Check sheet for the drawn part. Datum: minimum x, y, z corner. Units: mm. Round coordinates to 2 decimals unless told otherwise and drop trailing zeros. Order: outer loops, then holes, each group sorted by start corner. A loop starts at its lowest first (then second) coordinate and runs counter-clockwise, first axis right, second up. Notation, with made-up numbers: (82, 66) - (140, 66) arc R17 cw to (140, 76) - close; hole circle Ø10 at (77.25, 84). An arc over 180 degrees is marked (long way). Write each question's results on one line, items separated by ' | '.
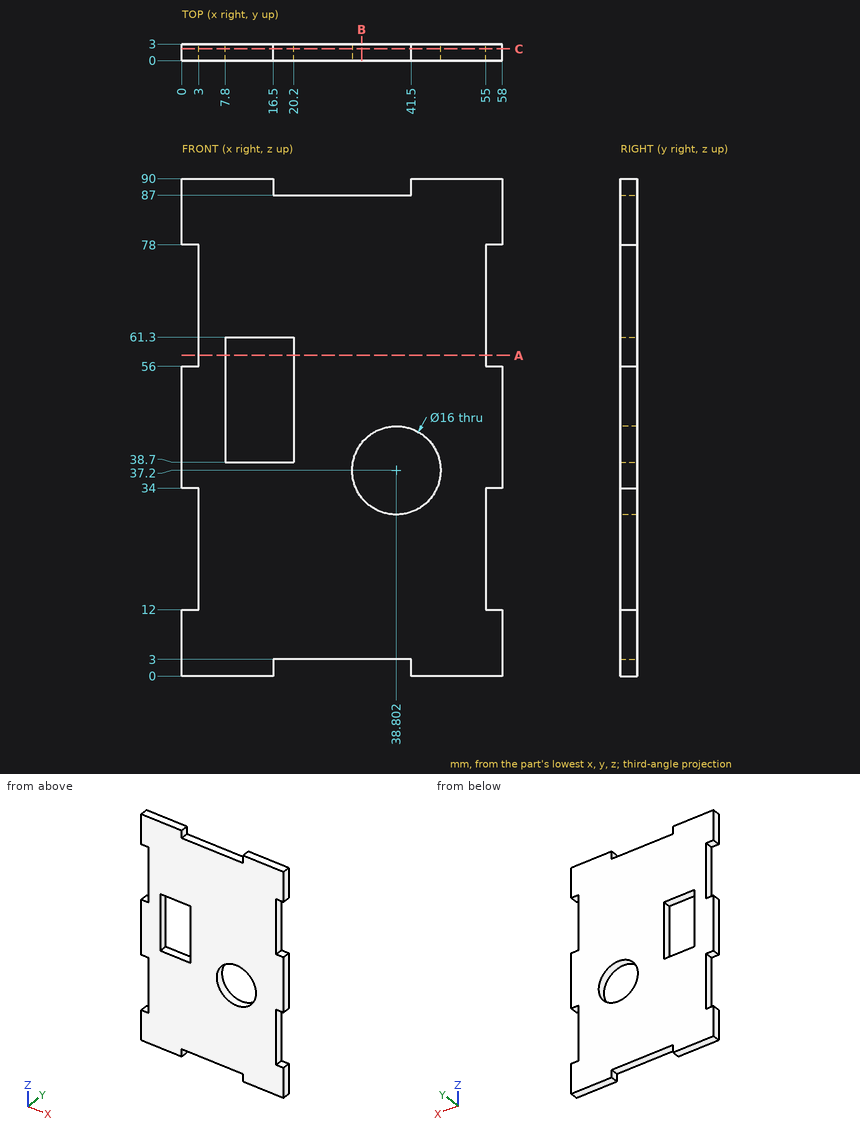
(1) Depth check by flat-ended pin: pin 1 Ø1 at (y, z) = (1.5, 23) entering from +X; pin 2 Ø0.9 at (y, z) = (2, 25.5) entering from -X. Enter the tip coordinate at first touch or a pass-through.
Answers follow:
pin 1: x = 55 | pin 2: x = 3
(2) Section check C-C (y = 2.1). Give the number of separate pieces and of enclosed holes in the cut face.
Answers follow:
separate pieces: 1 | enclosed holes: 2
(3) Section check A-A (z = 58). Record the cut outline in (x, y).
Answers follow:
outline: (3, 0) - (7.8, 0) - (7.8, 3) - (3, 3) - close; (20.2, 0) - (55, 0) - (55, 3) - (20.2, 3) - close
(4) Material ranges on line 1 (Z direction, x = 38.5, y = 0.25) (1 decimal); line 2 (X direction, y = 1.8, z = 46); line 3 (X direction, y = 1.1, z = 37.2), recorded low to high.
Answers follow:
line 1: 3 to 29.2, 45.2 to 87 | line 2: 0 to 7.8, 20.2 to 58 | line 3: 0 to 30.8, 46.8 to 58
(5) Section check B-B (x = 32.5). Record the cut outline in (y, z).
Answers follow:
outline: (0, 3) - (3, 3) - (3, 32.27) - (0, 32.27) - close; (0, 42.13) - (3, 42.13) - (3, 87) - (0, 87) - close
